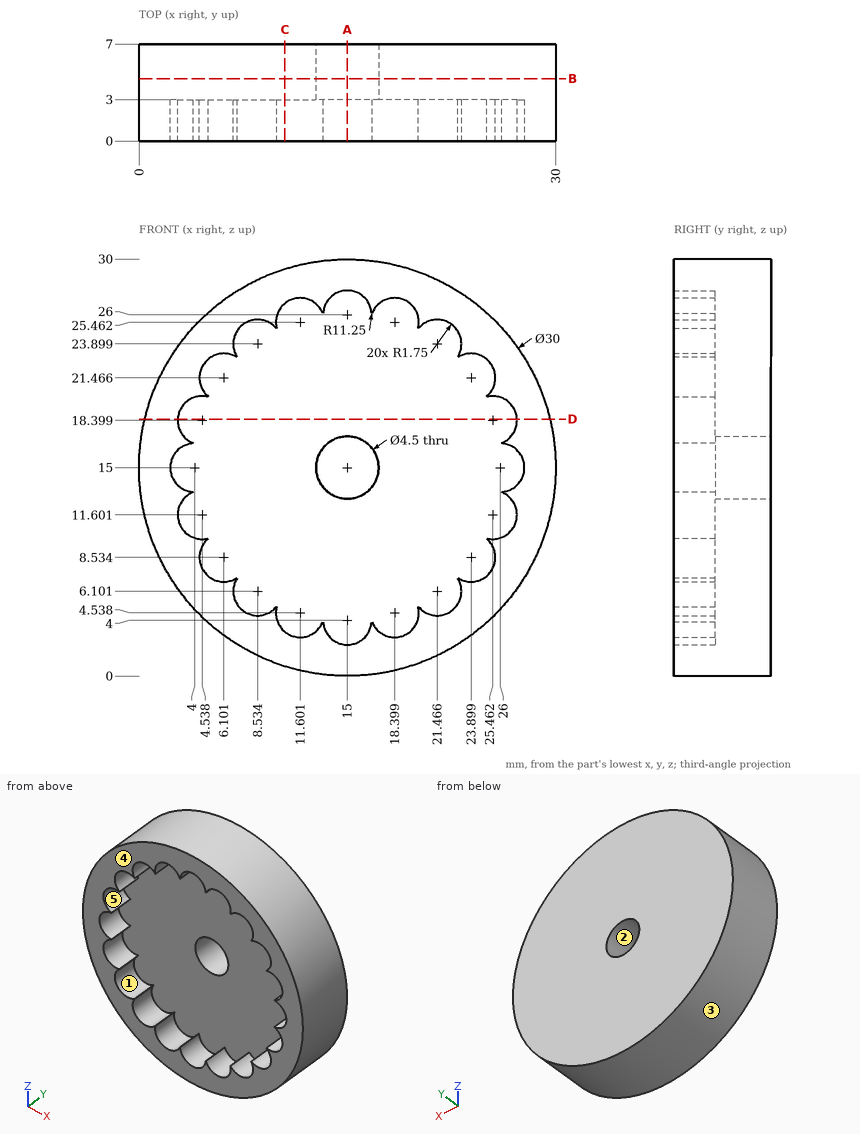
Part print with two shaded views. Sizes in mm from the minimum x, y, z corner. A direction names the side the tool comes from. Round coordinates to 2 decimals unless told otherwise and drop trailing zeros. Loops run counter-clockwise (first coordinate to the right, second up) from the corner with the lowest first, then second, coordinate; pieces in that order, holes last. Notation, with made-up numbers: (71.5, 12.25) - (94.5, 12.25) arc R12 cw to (94.5, 28.25) - close; hole circle Ø11 at (87, 45.25). An arc over 180 degrees is marked (long way). Answer as a JSON object with one key per item and string values.
Item 1: Band-saw the part on D-D on z = 18.5. List the corners of the cut face in (x, y).
Output:
{"outline": "(0.41, 0) - (2.79, 0) - (2.79, 3) - (27.21, 3) - (27.21, 0) - (29.59, 0) - (29.59, 7) - (0.41, 7) - close"}
Item 2: Band-saw the part on B-B on y = 4.5. List the corners of the cut face in (x, z), plus the area to 3 significant figures.
Output:
{"outline": "circle Ø30 at (15, 15); hole circle Ø4.5 at (15, 15)", "area": "691 mm2"}
Item 3: Pull direction X, two halves, no side cores. Call the marked faces 3, 4 and 5: pulls with the +X half, pulls with the -X half, needs draft (parallel to the pull), parting line crosses it, or undercut.
Output:
{"face 3": "parting line crosses it", "face 4": "needs draft", "face 5": "undercut"}
Item 4: Pin check, flat tips, straight feed: pin 1 (3 mm diameter, centred on x = 19, y = 3, fed in from +Z); pin 2 (1.5 mm diameter, centred on x = 23, y = 1.5, fed in from +Z). Stop position of each tip, or through.
Output:
{"pin 1": "z = 29.79", "pin 2": "z = 28.13"}
Item 5: Tool access for the marked faces 1 and 2: list every direction of +Z, -Z, +X, -X, +Y, -Y with a clear straight run to the whole face (end or side of a thin tool).
Output:
{"face 1": "-Y", "face 2": "+Y, -Y"}
Item 6: Band-saw the part on C-C on x = 10.5. List the corners of the cut face in (y, z), plus the area to 3 significant figures.
Output:
{"outline": "(0, 0.69) - (7, 0.69) - (7, 29.31) - (0, 29.31) - (0, 26.82) - (3, 26.82) - (3, 3.18) - (0, 3.18) - close", "area": "129 mm2"}
Item 7: Wall check: L1, parallel to Z at x = 15, y = 4.35; L2, parallel to Y at x = 10.25, z = 19; L3, parallel to Z at x = 26, y = 1.5 (1 decimal). Give the ranges that are in metal, low to high.
Output:
{"L1": "0 to 12.75, 17.25 to 30", "L2": "3 to 7", "L3": "4.8 to 9.9, 20.1 to 25.2"}
Item 8: Band-saw the part on A-A on x = 15. List the corners of the cut face in (y, z).
Output:
{"outline": "(0, 0) - (7, 0) - (7, 12.75) - (3, 12.75) - (3, 2.25) - (0, 2.25) - close; (0, 27.75) - (3, 27.75) - (3, 17.25) - (7, 17.25) - (7, 30) - (0, 30) - close"}
